from build123d import *

# Parameters (mm, degrees)
SKETCH1_W           = 40
SKETCH1_H           = 17
BOSS_EXTRUDE1_DEPTH = 1.4
CUT_EXTRUDE1_START  = 1.4
SKETCH3_W           = 16
SKETCH3_H           = 4
SKETCH3_W_2         = 3
SKETCH3_H_2         = 11
CUT_EXTRUDE1_DEPTH  = 1
SKETCH4_R           = 1.3
CUT_EXTRUDE2_DEPTH  = 11
SKETCH7_W           = 9
SKETCH7_H           = 17
CUT_EXTRUDE5_DEPTH  = 21
SKETCH9_R           = 2.55
BOSS_EXTRUDE3_DEPTH = 3
FILLET2_R           = 10


with BuildPart() as part:
    # Sketch1 → Boss-Extrude1 (new body)
    with BuildSketch(Plane.XY):
        Rectangle(SKETCH1_W, SKETCH1_H)
    extrude(amount=BOSS_EXTRUDE1_DEPTH)

    # Sketch3 → Cut-Extrude1 (cut)
    with BuildSketch(Plane.XY.offset(CUT_EXTRUDE1_START)):
        with Locations((7, -1)):
            Rectangle(SKETCH3_W, SKETCH3_H)
        with Locations((-9.5, -1)):
            Rectangle(SKETCH3_W_2, SKETCH3_H_2)
    extrude(amount=-CUT_EXTRUDE1_DEPTH, mode=Mode.SUBTRACT)

    # Sketch4 → Cut-Extrude2 (cut)
    with BuildSketch(Plane.XY):
        with Locations(Location((16, 5, 0), (0, 0, 180))):
            Circle(SKETCH4_R)
        with Locations(Location((-3, 5, 0), (0, 0, 180))):
            Circle(SKETCH4_R)
    extrude(amount=CUT_EXTRUDE2_DEPTH, mode=Mode.SUBTRACT)

    # Sketch7 → Cut-Extrude5 (cut)
    with BuildSketch(Plane.XY):
        with Locations((-15.5, 0)):
            Rectangle(SKETCH7_W, SKETCH7_H)
    extrude(amount=CUT_EXTRUDE5_DEPTH, mode=Mode.SUBTRACT)

    # Sketch9 → Boss-Extrude3 (add)
    with BuildSketch(Plane.XY):
        Polygon((-12, -8.5), (-12, -28.5), (4, -28.5), (4, -8.5), (-4, -8.5), align=None)
        with Locations((-4, -13)):
            Circle(SKETCH9_R, mode=Mode.SUBTRACT)
        with Locations((-4, -24)):
            Circle(SKETCH9_R, mode=Mode.SUBTRACT)
    extrude(amount=BOSS_EXTRUDE3_DEPTH)

    # Fillet2
    # the kernel refuses this fillet: 10 mm, written as the material it adds along each edge
    with BuildSketch(Plane(origin=(-11, -8.5, 0), x_dir=(0, 1, 0), z_dir=(0, 0, 1))) as fillet2_piece_1_section:
        with BuildLine():
            CenterArc((4.358898944, 10), FILLET2_R, 244.158067237, 25.841932763)
            Line((0, 1), (0, 0))
            Line((0, 0), (4.358898944, 0))
        make_face()
    fillet2_piece_1 = extrude(amount=12.297247359, mode=Mode.PRIVATE)
    fillet2_piece_1 = split(fillet2_piece_1, bisect_by=Plane(origin=(-11, -8.5, 0.4), z_dir=(0, 0, -1)), keep=Keep.TOP, mode=Mode.PRIVATE)
    add(fillet2_piece_1)
    with BuildSketch(Plane(origin=(-11, -8.5, -10.897247359), x_dir=(0, 1, 0), z_dir=(0, 0, 1))) as fillet2_piece_2_section:
        with BuildLine():
            CenterArc((4.358898944, 10), FILLET2_R, 244.158067237, 25.841932763)
            Line((0, 1), (0, 0))
            Line((0, 0), (4.358898944, 0))
        make_face()
    fillet2_piece_2 = extrude(amount=12.297247359, mode=Mode.PRIVATE)
    fillet2_piece_2 = split(fillet2_piece_2, bisect_by=Plane(origin=(-11, -6.5, -10.897247359), z_dir=(0, -1, 0)), keep=Keep.TOP, mode=Mode.PRIVATE)
    fillet2_piece_2 = split(fillet2_piece_2, bisect_by=Plane(origin=(-11, -8.5, 0.4), z_dir=(0, 0, 1)), keep=Keep.TOP, mode=Mode.PRIVATE)
    add(fillet2_piece_2)
    with BuildSketch(Plane(origin=(4, -8.5, 0), x_dir=(1, 0, 0), z_dir=(0, 0, 1))) as fillet2_piece_3:
        with BuildLine():
            CenterArc((FILLET2_R, -FILLET2_R), FILLET2_R, 90, 90)
            Line((0, -FILLET2_R), (0, 0))
            Line((0, 0), (FILLET2_R, 0))
        make_face()
    extrude(amount=1.4)


solid = part.part
CAD build for the part. Positions are in the model's coordinates, mm. A direction names the side the tool comes from. Round coordinates to 2 decimals unless told otherwise and drop trailing zeros. Order: outer loops, then holes, each group sorted by start corner. A loop starts at its lowest first (then second) coordinate and runs counter-clockwise, first axis right, second up. Notation, with made-up numbers: (40, 12) -> (92, 12) arc R8 ccw to (92, 24) -> close; hole circle Ø9 at (38.25, 79.5). An arc over 180 degrees is marked (long way). Write item = value, one per line. Start each with the question number.
(1) Which spindle directions (+Z, -Z, +X, -X, +Y, -Y) get a long thin tool onto all of the face, cutting with end or side? Do faces 4 (the flat face through (-8, -1, 1)), 5 (the flat face through (-11, 3.5, 0.2)), 6 (the flat face through (15, -1, 1)). Say none if no direction does.
(2) Probe line 1 (X direction, y = 5, z = 0.6); line 2 (Y direction, x = -4, z = 2.4); line 3 (Y direction, x = 19.5, z = 0.65). List the from-to ranges inside material, lowest first. Write a range as [from, to].
(3) Cut at D-D, the plane x = 8. List the corners of the cut face in (y, z), then the cut area to 3 significant figures.
(4) Pull direction X, two halves, no side cores. Call faces 1 (the flat face through (4, -21, 2)), 2 (the flat face through (-4, -8.5, 2)), 3 (the cylindrical face through (-2.72, 6.27, 0.69)): released by +X, released by -X, zero draft, split by the parting line, or undercut.
(5) Cut at B-B, the plane y = 5. List the corners of the cut face in (x, z).
(6) Pin check, flat tips, straight feed: P1, Ø1, axis at y = -1, z = 1, coming from the -X side; P2, Ø5, axis at x = 3.5, y = -16, coming from the -Z side; P3, Ø1.6, axis at x = -9.5, y = -3, coming from the +Z side; P4, Ø1.1, axis at y = 5, z = 0.5, coming from the -X side. Stop position of each tip, or through.
(7) Cut at A-A, the plane x = 16. List the corners of the cut face in (y, z), then the cut area to 3 significant figures.
(8) Cut at C-C, the plane y = -14.5. List the corners of the cut face in (x, z), then the cut area to 3 significant figures.
Model answer:
q1.face_4 = +Z, -X
q1.face_5 = +Z, -Z, -X, +Y
q1.face_6 = +Z
q2.line_1 = [-11, -4.3], [-1.7, 14.7], [17.3, 20]
q2.line_2 = [-28.5, -26.55], [-21.45, -15.55], [-10.45, -8.5]
q2.line_3 = [-8.5, 8.5]
q3.outline = (-10.5, 0) -> (8.5, 0) -> (8.5, 1.4) -> (1, 1.4) -> (1, 0.4) -> (-3, 0.4) -> (-3, 1.4) -> (-10.5, 1.4) -> close
q3.area = 22.6 mm2
q4.face_1 = released by +X
q4.face_2 = zero draft
q4.face_3 = undercut
q5.outline = (-11, 0) -> (-4.3, 0) -> (-4.3, 1.4) -> (-11, 1.4) -> close; (-1.7, 0) -> (14.7, 0) -> (14.7, 1.4) -> (-1.7, 1.4) -> close; (17.3, 0) -> (20, 0) -> (20, 1.4) -> (17.3, 1.4) -> close
q6.P1 = -8
q6.P2 = 0
q6.P3 = 0.4
q6.P4 = -11
q7.outline = (-8.5, 0) -> (3.7, 0) -> (3.7, 1.4) -> (-8.5, 1.4) -> close; (6.3, 0) -> (8.5, 0) -> (8.5, 1.4) -> (6.3, 1.4) -> close
q7.area = 20.2 mm2
q8.outline = (-12, 0) -> (-6.06, 0) -> (-6.06, 3) -> (-12, 3) -> close; (-1.94, 0) -> (4.83, 0) -> (4.83, 1.4) -> (4, 1.4) -> (4, 3) -> (-1.94, 3) -> close
q8.area = 36.8 mm2
